For this review, use the dimensioned drawing (mm, ordinates from the lowest corner) and the shaded views. Coordinates: 2 decimals unless noted, no trailing zeros. Loops run counter-clockwise (first coordinate to the right, second up) from the corner with the lowest first, then second, coordinate; pieces in that order, holes last. Notation, with made-up numbers: (82.5, -20) - (96.5, -20) arc R28 ccw to (96.5, -2) - close; hole circle Ø10 at (56.5, 55). An arc over 180 degrees is marked (long way). Return JSON: item names as keys, results as strings. Group by question number.
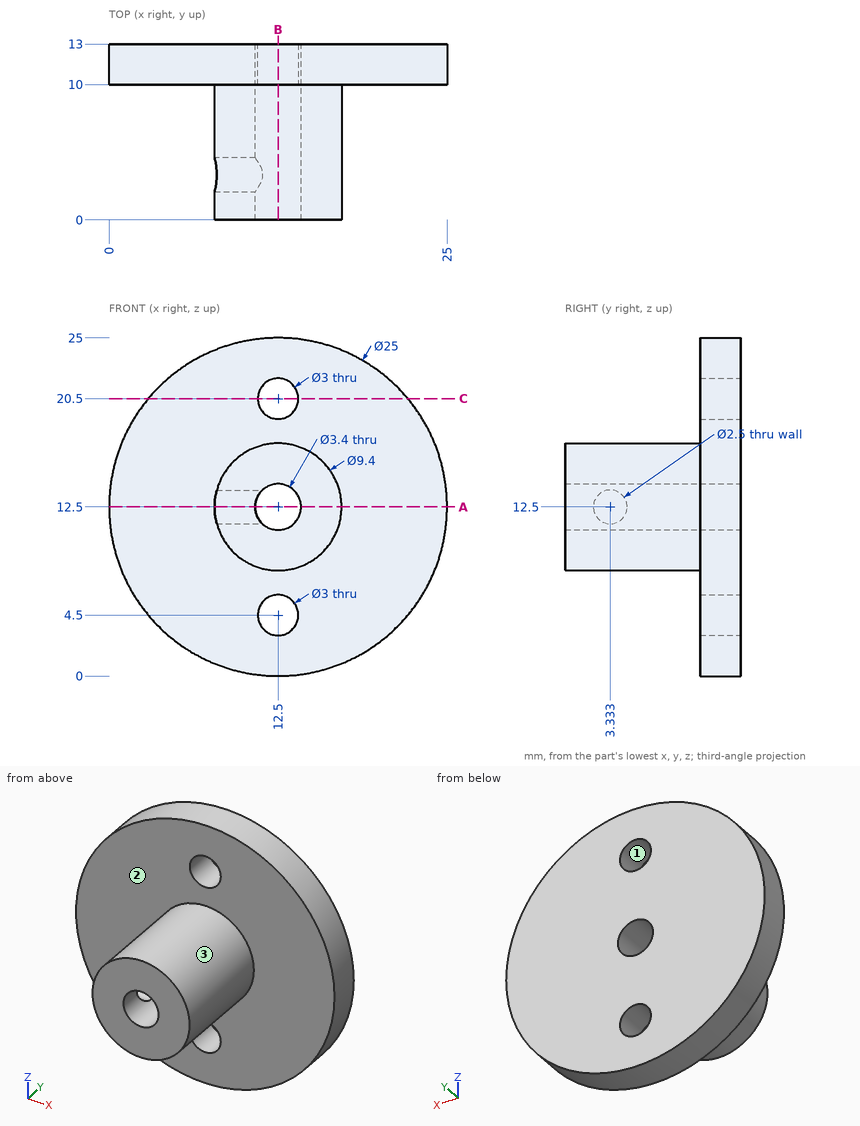
Item 1: Add section A-A (z = 12.5). State the section outline as (x, y) points.
Item 2: For P1, Ø1.5, axis at y = 3.33, z = 12.5, coming from the +X side; P2, Ø3, axis at x = 13, y = 3, coming from the -Z side; P3, Ø1.5, axis at y = 8, z = 13.5, coming from the -X side; P4, Ø4, axis at y = 2, z = 4, coming from the +X side, all flat-tipped, find the tip position at first contact; note any pin that passes through.
Item 3: Draft analysis for pull direction Z (two halves, no side actions). For the marked faces 1, 2 and 3, state which applies: pulls with the +Z half, pulls with the -Z half, needs draft (parallel to the pull), parting line crosses it, or undercut.
Item 4: Add section C-C (z = 20.5). State the section outline as (x, y) points (1 decimal).
Item 5: Add section B-B (x = 12.5). State the section outline as (y, z) points, then the cut area to 3 significant figures.
Item 6: To check wall thickness, follow line 1 (Z direction, x = 12.5, y = 10.25); line 2 (Y direction, x = 17.5, z = 16.5); line 3 (X direction, y = 10.25, z = 21.5) (1 decimal). State the ranges of each line that lie inside material, in increasing order. Write a range as from..to.
Answers below:
{
 "1": {"outline": "(0, 10) - (7.8, 10) - (7.8, 4.58) - (10.8, 4.58) - (10.8, 13) - (0, 13) - close; (7.8, 0) - (10.8, 0) - (10.8, 2.08) - (7.8, 2.08) - close; (14.2, 0) - (17.2, 0) - (17.2, 10) - (25, 10) - (25, 13) - (14.2, 13) - close"},
 "2": {"P1": "stops at x = 17.2", "P2": "stops at z = 7.8", "P3": "stops at x = 7.81", "P4": "passes through"},
 "3": {"face 1": "undercut", "face 2": "needs draft", "face 3": "parting line crosses it"},
 "4": {"outline": "(2.9, 10) - (11, 10) - (11, 13) - (2.9, 13) - close; (14, 10) - (22.1, 10) - (22.1, 13) - (14, 13) - close"},
 "5": {"outline": "(0, 7.8) - (10, 7.8) - (10, 6) - (13, 6) - (13, 10.8) - (0, 10.8) - close; (0, 14.2) - (13, 14.2) - (13, 19) - (10, 19) - (10, 17.2) - (0, 17.2) - close; (10, 0) - (13, 0) - (13, 3) - (10, 3) - close; (10, 22) - (13, 22) - (13, 25) - (10, 25) - close", "area": "107 mm^2"},
 "6": {"line 1": "z = 0..3, 6..10.8, 14.2..19, 22..25", "line 2": "y = 10..13", "line 3": "x = 3.8..11.4, 13.6..21.2"}
}
